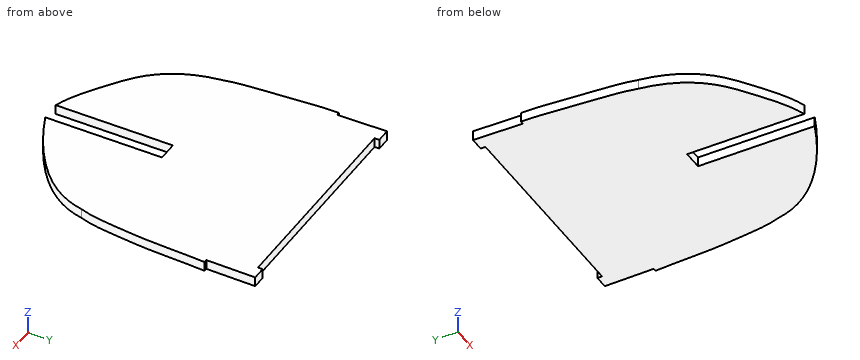
from build123d import *

# Parameters (mm, degrees)
EXTRUDE_1_DEPTH = 4


with BuildPart() as part:
    # 草图1 → 凸台-拉伸1 (new body)
    with BuildSketch(Plane.XY):
        with BuildLine():
            Line((192.01570903, 236.215172683), (197.691755822, 236.215172683))
            Line((197.691755822, 236.215172683), (197.691755822, 234.272114968))
            Line((197.691755822, 234.272114968), (283.716181534, 234.272114968))
            Line((283.716181534, 234.272114968), (283.716181534, 236.215172683))
            Line((283.716181534, 236.215172683), (289.16648845, 236.215172683))
            Line((289.16648845, 236.215172683), (288.899951815, 215.97975226))
            Line((288.899951815, 215.97975226), (290.208767161, 215.97975226))
            add(Edge.make_bspline(
                [(284.799620172, 162.392429744), (286.759474849, 167.893462355), (287.57993928, 177.029821997), (289.649811574, 194.897723767), (289.52739364, 207.149942748), (290.208767161, 215.97975226)],
                knots=[0, 0, 0, 0, 0.321928336, 0.507408205, 1, 1, 1, 1], degree=3))
            add(Edge.make_bspline(
                [(244.559945218, 125.200650029), (246.510897062, 126.005562495), (253.842274844, 129.235901905), (270.285883988, 138.599536344), (282.598559802, 151.178754354), (284.799620172, 162.392429744)],
                knots=[0.030116407, 0.030116407, 0.030116407, 0.030116407, 0.138264507, 0.441021692, 1, 1, 1, 1], degree=3))
            Line((244.559945218, 125.200650029), (244.559945218, 169.113949314))
            Line((244.559945218, 169.113949314), (244.559945218, 173.113949314))
            Line((244.559945218, 173.113949314), (236.559945217, 173.113949314))
            Line((236.559945217, 173.113949314), (236.559945217, 169.113949314))
            Line((236.559945217, 169.113949314), (236.559945217, 125.032675044))
            add(Edge.make_bspline(
                [(194.814526021, 169.905399038), (195.610141371, 164.176898927), (198.346571661, 154.492253984), (207.021687023, 142.787448402), (216.390436057, 136.399663861), (225.951903337, 129.821011624), (232.271114311, 126.432484596), (236.559945217, 125.032675044)],
                knots=[0, 0, 0, 0, 0.262954959, 0.448389479, 0.647828965, 0.773904026, 0.974785001, 0.974785001, 0.974785001, 0.974785001], degree=3))
            add(Edge.make_bspline(
                [(191.044749595, 215.97975226), (190.906681757, 208.303976986), (192.789425639, 192.9807794), (193.135017556, 177.533691326), (194.814526021, 169.905399038)],
                knots=[0, 0, 0, 0, 0.496472492, 1, 1, 1, 1], degree=3))
            Line((191.044749595, 215.97975226), (192.397258047, 215.97975226))
            Line((192.397258047, 215.97975226), (192.01570903, 236.215172683))
        make_face()
    extrude(amount=EXTRUDE_1_DEPTH)


solid = part.part
For this review, take the finished solid that the model builds, in its own axes (mm). Give positions to 0.01 mm unless a question says otherwise; leave off trailing zeros. Loops run counter-clockwise (first coordinate to the right, second up) from the corner with the lowest first, then second, coordinate; pieces in that order, holes last. Notation, with made-up numbers: M -40,22.5 L -34,22.5 A20 cw -34,26.5 Z; hole C 21.5,39.5 d1. An arc over 180 degrees is marked long. Answer as a JSON object with one key per item and string values. Group by question number.
Q1. For probe 1 along Y at (x, z) = (236.5, 3.5); probe 2 along X at (y, z) = (165, 3.5); probe 3 along X at (y, z) = (162, 3), list the stretches that pass through material, from the lowest coordinate up. Write a range as [from, to].
Q2. Insertion check: P1, Ø1.2, axis at y = 149.5, z = 2.5, coming from the +X side; P2, Ø0.6, axis at y = 235, z = 2, coming from the -X side; P3, Ø2, axis at x = 235, z = 1.5, coming from the +Y side. Each pin has a flat end and moves straight along its axis. Give the tip position at first contact, or say it passes through.
Q3. Add section A-A on x = 238.5. Give the boundary of the cut face in (y, z), and give its area (3 significant figures).
Checked values:
{
 "1": {"probe 1": "[125.05, 234.27]", "probe 2": "[195.71, 236.56], [244.56, 285.62]", "probe 3": "[196.48, 236.56], [244.56, 284.72]"},
 "2": {"P1": "x = 279.54", "P2": "x = 192.03", "P3": "y = 234.27"},
 "3": {"outline": "M 173.11,0 L 234.27,0 L 234.27,4 L 173.11,4 Z", "area": "245 mm²"}
}
